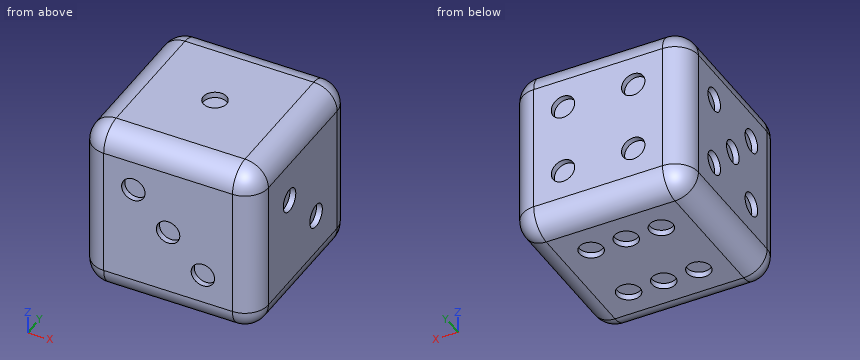
from build123d import *

# Parameters (mm, degrees)
F0_W      = 15
F0_H      = 15
F1_DEPTH  = 15
F2_R      = 2
F3_R      = 1
F4_DEPTH  = 0.5
F5_R      = 1
F6_DEPTH  = 0.5
F7_R      = 1
F8_DEPTH  = 0.5
F9_R      = 1
F10_DEPTH = 0.5
F11_R     = 1
F12_DEPTH = 0.5
F13_R     = 1
F14_DEPTH = 0.5


with BuildPart() as f1:
    # F0 (on Top) → F1 (new body)
    with BuildSketch(Plane.XY):
        with Locations((-7.5, 7.5)):
            Rectangle(F0_W, F0_H)
    extrude(amount=F1_DEPTH)

    # F2
    f2_edges = [f1.edges().sort_by_distance(p)[0] for p in [
        (-15, 15, 7.5),
        (0, 15, 7.5),
        (0, 0, 7.5),
        (-7.5, 0, 15),
        (-7.5, 15, 0),
        (-7.5, 15, 15),
        (-15, 0, 7.5),
        (-7.5, 0, 0),
        (0, 7.5, 0),
        (0, 7.5, 15),
        (-15, 7.5, 0),
        (-15, 7.5, 15),
    ]]
    fillet(f2_edges, radius=F2_R)

    # F3 (on face) → F4 (cut)
    with BuildSketch(Plane.XY.offset(15)):
        with Locations((-7.5, 7.5)):
            Circle(F3_R)
    extrude(amount=-F4_DEPTH, mode=Mode.SUBTRACT)

    # F5 (on face) → F6 (cut)
    with BuildSketch(Plane(origin=(0, 0, 0), x_dir=(1, 0, 0), z_dir=(0, 0, -1))):
        with Locations((-4.5, -10.5)):
            Circle(F5_R)
        with Locations((-7.5, -10.5)):
            Circle(F5_R)
        with Locations((-10.5, -10.5)):
            Circle(F5_R)
        with Locations((-10.5, -4.5)):
            Circle(F5_R)
        with Locations((-7.5, -4.5)):
            Circle(F5_R)
        with Locations((-4.5, -4.5)):
            Circle(F5_R)
    extrude(amount=-F6_DEPTH, mode=Mode.SUBTRACT)

    # F7 (on face) → F8 (cut)
    with BuildSketch(Plane(origin=(0, 15, 0), x_dir=(-1, 0, 0), z_dir=(0, 1, 0))):
        with Locations((10.5, 10.5)):
            Circle(F7_R)
        with Locations((4.5, 10.5)):
            Circle(F7_R)
        with Locations((4.5, 4.5)):
            Circle(F7_R)
        with Locations((10.5, 4.5)):
            Circle(F7_R)
    extrude(amount=-F8_DEPTH, mode=Mode.SUBTRACT)

    # F9 (on face) → F10 (cut)
    with BuildSketch(Plane.XZ):
        with Locations((-10.469848, 10.469848)):
            Circle(F9_R)
        with Locations((-7.5, 7.5)):
            Circle(F9_R)
        with Locations((-4.530152, 4.530152)):
            Circle(F9_R)
    extrude(amount=-F10_DEPTH, mode=Mode.SUBTRACT)

    # F11 (on face) → F12 (cut)
    with BuildSketch(Plane.YZ):
        with Locations((5.37868, 9.62132)):
            Circle(F11_R)
        with Locations((9.62132, 5.37868)):
            Circle(F11_R)
    extrude(amount=-F12_DEPTH, mode=Mode.SUBTRACT)

    # F13 (on face) → F14 (cut)
    with BuildSketch(Plane(origin=(-15, 0, 0), x_dir=(0, -1, 0), z_dir=(-1, 0, 0))):
        with Locations((-10.469848, 10.469848)):
            Circle(F13_R)
        with Locations((-4.530152, 10.469848)):
            Circle(F13_R)
        with Locations((-7.5, 7.5)):
            Circle(F13_R)
        with Locations((-10.469848, 4.530152)):
            Circle(F13_R)
        with Locations((-4.530152, 4.530152)):
            Circle(F13_R)
    extrude(amount=-F14_DEPTH, mode=Mode.SUBTRACT)


solid = f1.part
Verification items for the finished model (mm, model axes). Coordinates: 2 decimals unless noted, no trailing zeros. Write each loop counter-clockwise with the first axis right and the second up, starting at its lowest first coordinate (ties: lowest second). Pieces come first, ordered by that corner, then holes. Notation, with made-up numbers: M 22.5,-10 L 79.5,-10 A21 cw 79.5,6 Z; hole C -35.75,57 d1. An arc over 180 degrees is marked long. Use a Markdown table: item, result.
Q1. Thickness scan on line 1 (Y direction, x = -7.5, z = 0.2); line 2 (Z direction, x = -4.5, y = 14.75); line 3 (X direction, y = 10, z = 9.75). Record the ranges inside material, lowest first.
Reply:
| item | result |
|---|---|
| line 1 | y = 1.13 to 3.5, 5.5 to 9.5, 11.5 to 13.87 |
| line 2 | z = 1.03 to 3.5, 5.5 to 9.5, 11.5 to 13.97 |
| line 3 | x = -14.5 to 0 |
Q2. Sectioned sample at B-B, the plane x = -7.5. Record the boundary of the cut face in (y, z).
Reply:
| item | result |
|---|---|
| outline | M 0,2 A2 ccw 2,0 L 3.5,0 L 3.5,0.5 L 5.5,0.5 L 5.5,0 L 9.5,0 L 9.5,0.5 L 11.5,0.5 L 11.5,0 L 13,0 A2 ccw 15,2 L 15,13 A2 ccw 13,15 L 8.5,15 L 8.5,14.5 L 6.5,14.5 L 6.5,15 L 2,15 A2 ccw 0,13 L 0,8.5 L 0.5,8.5 L 0.5,6.5 L 0,6.5 Z |
Q3. Sectioned sample at D-D, the plane x = -4.5. Record the boundary of the cut face in (y, z).
Reply:
| item | result |
|---|---|
| outline | M 0,2 A2 ccw 2,0 L 3.5,0 L 3.5,0.5 L 5.5,0.5 L 5.5,0 L 9.5,0 L 9.5,0.5 L 11.5,0.5 L 11.5,0 L 13,0 A2 ccw 15,2 L 15,3.5 L 14.5,3.5 L 14.5,5.5 L 15,5.5 L 15,9.5 L 14.5,9.5 L 14.5,11.5 L 15,11.5 L 15,13 A2 ccw 13,15 L 2,15 A2 ccw 0,13 L 0,5.53 L 0.5,5.53 L 0.5,3.53 L 0,3.53 Z |
Q4. Sectioned sample at C-C, the plane z = 7. Record the boundary of the cut face in (x, y).
Reply:
| item | result |
|---|---|
| outline | M -15,2 A2 ccw -13,0 L -8.37,0 L -8.37,0.5 L -6.63,0.5 L -6.63,0 L -2,0 A2 ccw 0,2 L 0,13 A2 ccw -2,15 L -13,15 A2 ccw -15,13 L -15,8.37 L -14.5,8.37 L -14.5,6.63 L -15,6.63 Z |
Q5. Sectioned sample at A-A, the plane y = 7.5. Record the boundary of the cut face in (x, z), plus the area to 3 significant figures.
Reply:
| item | result |
|---|---|
| outline | M -15,2 A2 ccw -13,0 L -2,0 A2 ccw 0,2 L 0,13 A2 ccw -2,15 L -6.5,15 L -6.5,14.5 L -8.5,14.5 L -8.5,15 L -13,15 A2 ccw -15,13 L -15,8.5 L -14.5,8.5 L -14.5,6.5 L -15,6.5 Z |
| area | 220 mm² |
Q6. Go/stop test with flat-tipped pins: P1, Ø1.6, axis at x = -7.5, y = 7.5, coming from the +Z side; P2, Ø0.6, axis at x = -10.5, z = 11, coming from the -Y side; P3, Ø0.6, axis at x = -4.5, z = 10, coming from the +Y side. Record where each tip stops, or that it passes through.
Reply:
| item | result |
|---|---|
| P1 | stops at z = 14.5 |
| P2 | stops at y = 0.5 |
| P3 | stops at y = 14.5 |
